Input: part model. Units: mm. Frame: model coordinates. A direction names the side the tool comes from. Give positions to 0.01 mm unless a question says otherwise; leave off trailing zeros. Loops run counter-clockwise (first coordinate to the right, second up) from the corner with the lowest first, then second, coordinate; pieces in that order, holes last. Notation, with made-up numbers: M 25.5,69 L 49.5,69 A27 cw 49.5,104 Z; hole C 9,-21 d11. An arc over 180 degrees is marked long. Answer as a JSON object with one key per item and string values. Group by question number.
```python
from build123d import *

# Parameters (mm, degrees)
SKETCH_1_W      = 87.2
SKETCH_1_H      = 21
EXTRUDE_1_DEPTH = 1.7
SKETCH_2_W      = 79.2
SKETCH_2_H      = 16
EXTRUDE_2_DEPTH = 1.2
FILLET_1_R      = 3
FILLET_2_R      = 1


with BuildPart() as part:
    # Эскиз1 → Бобышка-Вытянуть1 (new body)
    with BuildSketch(Plane.XY):
        Rectangle(SKETCH_1_W, SKETCH_1_H)
    extrude(amount=EXTRUDE_1_DEPTH)

    # Эскиз2 → Бобышка-Вытянуть2 (add)
    with BuildSketch(Plane.XY.offset(1.7)):
        Rectangle(SKETCH_2_W, SKETCH_2_H)
    extrude(amount=EXTRUDE_2_DEPTH)

    # Скругление1
    fillet_1_edges = [part.edges().sort_by_distance(p)[0] for p in [
        (39.6, -8, 2.3),
        (39.6, 8, 2.3),
        (-39.6, 8, 2.3),
        (-39.6, -8, 2.3),
    ]]
    fillet(fillet_1_edges, radius=FILLET_1_R)

    # Скругление2
    fillet_2_edges = [part.edges().sort_by_distance(p)[0] for p in [
        (43.6, -10.5, 0.85),
        (-43.6, -10.5, 0.85),
        (-43.6, 10.5, 0.85),
        (43.6, 10.5, 0.85),
    ]]
    fillet(fillet_2_edges, radius=FILLET_2_R)


solid = part.part
```
1. First-contact query: P1, Ø1.3, axis at y = -0.5, z = 2.5, coming from the +X side; P2, Ø0.6, axis at x = -5, z = 2.5, coming from the +Y side; P3, Ø0.6, axis at y = 0, z = 2.5, coming from the -X side. Flat tips, straight axial feed; report the tip coordinate or a pass-through.
2. Section A-A (y = 3.25). Output: boundary loops of the cut face in (x, z).
3. Section B-B (x = -32.5). Output: boundary loops of the cut face in (y, z), then the cut area to 3 significant figures.
4. Material intervals for L1, parallel to X at y = 4.75, z = 2.3; L2, parallel to Z at x = -34, y = -8.75; L3, parallel to Y at x = 20.5, z = 2.3, sorted ascending.
5. Reachability of faces 1 (the cylindrical face through (-38.7, -7.14, 2.31)), 2 (the cylindrical face through (-38.7, 7.14, 2.31)), 3 (the cylindrical face through (38.74, 7.1, 2.31)), 4 (the cylindrical face through (38.7, -7.14, 2.31)), 5 (the flat face through (-1, 0, 2.9)) from +Z, -Z, +X, -X, +Y, -Y: full face, straight path, thin tool, end or side. Return the list, or none.
Geometry results:
{
 "1": {"P1": "x = 39.6", "P2": "y = 8", "P3": "x = -39.6"},
 "2": {"outline": "M -43.6,0 L 43.6,0 L 43.6,1.7 L 39.6,1.7 L 39.6,2.9 L -39.6,2.9 L -39.6,1.7 L -43.6,1.7 Z"},
 "3": {"outline": "M -10.5,0 L 10.5,0 L 10.5,1.7 L 8,1.7 L 8,2.9 L -8,2.9 L -8,1.7 L -10.5,1.7 Z", "area": "54.9 mm2"},
 "4": {"L1": "-39.6 to 39.6", "L2": "0 to 1.7", "L3": "-8 to 8"},
 "5": {"face 1": "+Z, -X, -Y", "face 2": "+Z, -X, +Y", "face 3": "+Z, +X, +Y", "face 4": "+Z, +X, -Y", "face 5": "+Z, +X, -X, +Y, -Y"}
}
